Geometry: final body of the model. Coordinates: model frame, mm. A direction names the side the tool comes from. Give positions to 0.01 mm unless a question says otherwise; leave off trailing zeros. Order: outer loops, then holes, each group sorted by start corner. A loop starts at its lowest first (then second) coordinate and runs counter-clockwise, first axis right, second up. Notation, with made-up numbers: (39.5, 18) -> (44.5, 18) arc R7 cw to (44.5, 26) -> close; hole circle Ø10 at (-14, -27.5). An arc over 180 degrees is marked (long way). One line per question, with ' | ' between items.
from build123d import *

# Parameters (mm, degrees)
SKIZZE1_W                       = 64
SKIZZE1_H                       = 28
AUFSATZ_LINEAR_AUSTRAGEN1_DEPTH = 2
SKIZZE2_R                       = 1.75
SCHNITT_LINEAR_AUSTRAGEN1_DEPTH = 70.885620839
SKIZZE3_W                       = 2
SKIZZE3_H                       = 16
SCHNITT_LINEAR_AUSTRAGEN2_DEPTH = 70.885620839
LINEARES_MUSTER1_COUNT          = 4
LINEARES_MUSTER1_PITCH          = 4
SKIZZE5_W                       = 1.6
SKIZZE5_H                       = 10
SKIZZE5_W_2                     = 50
SKIZZE5_H_2                     = 1.6
SKIZZE5_W_3                     = 2
AUFSATZ_LINEAR_AUSTRAGEN2_DEPTH = 3
SKIZZE6_W                       = 52
SKIZZE6_H                       = 1.5
AUFSATZ_LINEAR_AUSTRAGEN3_DEPTH = 2
SKIZZE7_W                       = 56
SKIZZE7_H                       = 2.1
AUFSATZ_LINEAR_AUSTRAGEN4_DEPTH = 2
FASE1_SIZE2                     = 0.6
FASE1_SIZE                      = 2


with BuildPart() as part:
    # Skizze1 → Aufsatz-Linear austragen1 (new body)
    with BuildSketch(Plane(origin=(0, 0, 0), x_dir=(1, 0, 0), z_dir=(0, 1, 0))):
        with Locations((32, 14)):
            Rectangle(SKIZZE1_W, SKIZZE1_H)
    extrude(amount=AUFSATZ_LINEAR_AUSTRAGEN1_DEPTH)

    # Skizze2 → Schnitt-Linear austragen1 (cut, through all)
    with BuildSketch(Plane(origin=(0, 2, 0), x_dir=(1, 0, 0), z_dir=(0, 1, 0))):
        with Locations(Location((3, 3, 0), (0, 0, 270))):
            Circle(SKIZZE2_R)
        with Locations(Location((3, 20.9, 0), (0, 0, 270))):
            Circle(SKIZZE2_R)
        with Locations(Location((61, 20.9, 0), (0, 0, 270))):
            Circle(SKIZZE2_R)
        with Locations(Location((61, 3, 0), (0, 0, 270))):
            Circle(SKIZZE2_R)
    extrude(amount=-SCHNITT_LINEAR_AUSTRAGEN1_DEPTH, mode=Mode.SUBTRACT)

    # Skizze3 → Schnitt-Linear austragen2 (cut, through all)
    with BuildSketch(Plane(origin=(0, 2, 0), x_dir=(1, 0, 0), z_dir=(0, 1, 0))):
        with Locations((27, 14)):
            Rectangle(SKIZZE3_W, SKIZZE3_H)
    schnitt_linear_austragen2 = extrude(amount=-SCHNITT_LINEAR_AUSTRAGEN2_DEPTH, mode=Mode.SUBTRACT)

    # Lineares Muster1: Schnitt-Linear austragen2 ×4
    with Locations(*[(i * LINEARES_MUSTER1_PITCH, 0, 0) for i in range(1, LINEARES_MUSTER1_COUNT)]):
        add(schnitt_linear_austragen2, mode=Mode.SUBTRACT)

    # Skizze5 → Aufsatz-Linear austragen2 (add)
    with BuildSketch(Plane(origin=(0, 2, 0), x_dir=(1, 0, 0), z_dir=(0, 1, 0))):
        with Locations((2.8, 12)):
            Rectangle(SKIZZE5_W, SKIZZE5_H)
        with Locations((32, 2.8)):
            Rectangle(SKIZZE5_W_2, SKIZZE5_H_2)
        with Locations((61, 12)):
            Rectangle(SKIZZE5_W_3, SKIZZE5_H)
    extrude(amount=AUFSATZ_LINEAR_AUSTRAGEN2_DEPTH)

    # Skizze6 → Aufsatz-Linear austragen3 (add)
    with BuildSketch(Plane(origin=(0, 2, 0), x_dir=(1, 0, 0), z_dir=(0, 1, 0))):
        with Locations((32, 23.15)):
            Rectangle(SKIZZE6_W, SKIZZE6_H)
    extrude(amount=AUFSATZ_LINEAR_AUSTRAGEN3_DEPTH)

    # Skizze7 → Aufsatz-Linear austragen4 (add)
    with BuildSketch(Plane(origin=(0, 2, 0), x_dir=(1, 0, 0), z_dir=(0, 1, 0))):
        with Locations((32, 26.95)):
            Rectangle(SKIZZE7_W, SKIZZE7_H)
    extrude(amount=AUFSATZ_LINEAR_AUSTRAGEN4_DEPTH)

    # Fase1
    fase1_edges = [part.edges().sort_by_distance(p)[0] for p in [
        (32, 4, -25.9),
    ]]
    fase1_side = [part.faces().sort_by_distance(p)[0] for p in [
        (32, 3.988, -25.9),
    ]]
    chamfer(fase1_edges, length=FASE1_SIZE - 0.0001, length2=FASE1_SIZE2 - 0.0001, reference=fase1_side[0])  # a hair under: the kernel refuses the full size


solid = part.part
1) Section C-C on z = -20.9. Return loops of the section in (x, y), plus the area to 3 significant figures.
Check result:
outline: (0, 0) -> (1.25, 0) -> (1.25, 2) -> (0, 2) -> close; (4.75, 0) -> (26, 0) -> (26, 2) -> (4.75, 2) -> close; (28, 0) -> (30, 0) -> (30, 2) -> (28, 2) -> close; (32, 0) -> (34, 0) -> (34, 2) -> (32, 2) -> close; (36, 0) -> (38, 0) -> (38, 2) -> (36, 2) -> close; (40, 0) -> (59.25, 0) -> (59.25, 2) -> (40, 2) -> close; (62.75, 0) -> (64, 0) -> (64, 2) -> (62.75, 2) -> close | area: 98.0 mm^2
2) Material intervals for probe 1 along X at (y, z) = (1.35, -3); probe 2 along X at (y, z) = (1.85, -14); probe 3 along Z at (x, y) = (31, 2.5), sorted ascending. Write a range as from..to.
Check result:
probe 1: x = 0..1.25, 4.75..59.25, 62.75..64 | probe 2: x = 0..26, 28..30, 32..34, 36..38, 40..64 | probe 3: z = -28..-26.05, -23.9..-22.4, -3.6..-2
3) Section A-A on z = -9.5. Return loops of the section in (x, y).
Check result:
outline: (0, 0) -> (26, 0) -> (26, 2) -> (3.6, 2) -> (3.6, 5) -> (2, 5) -> (2, 2) -> (0, 2) -> close; (28, 0) -> (30, 0) -> (30, 2) -> (28, 2) -> close; (32, 0) -> (34, 0) -> (34, 2) -> (32, 2) -> close; (36, 0) -> (38, 0) -> (38, 2) -> (36, 2) -> close; (40, 0) -> (64, 0) -> (64, 2) -> (62, 2) -> (62, 5) -> (60, 5) -> (60, 2) -> (40, 2) -> close
4) Contact query for flat-ended pins moving along their axis: pin 1 Ø1.5 at (x, y) = (20.5, 3.5) entering from +Z; pin 2 Ø4.5 at (x, z) = (61, -3) entering from +Y; pin 3 Ø12 at (x, z) = (29, -15) entering from -Y; pin 4 Ø3 at (x, z) = (3, -20.9) entering from -Y. Output: stop coordinate, or through.
Check result:
pin 1: stops at z = -2 | pin 2: stops at y = 2 | pin 3: stops at y = 0 | pin 4: passes through
5) Section B-B on y = 1.1. Count the separate pieces of the cut face and the enclosed holes in it, plus the area to 3 significant figures.
Check result:
separate pieces: 1 | enclosed holes: 8 | area: 1,630 mm^2
6) Section D-D on x = 61. Return loops of the section in (y, z).
Check result:
outline: (0, -28) -> (2, -28) -> (2, -22.65) -> (0, -22.65) -> close; (0, -19.15) -> (2, -19.15) -> (2, -17) -> (5, -17) -> (5, -7) -> (2, -7) -> (2, -4.75) -> (0, -4.75) -> close; (0, -1.25) -> (2, -1.25) -> (2, 0) -> (0, 0) -> close
7) Pull-direction query (X, two-part tool) for faces 5 (the flat face through (2, 3, -12)), 6 (the flat face through (40, 1, -14)), 7 (the flat face through (31, 1, -6)), 8 (the flat face through (64, 1, -14)); classes: +X half, -X half, draft (parallel to the pull), parting line (faces both ways), or undercut.
Check result:
face 5: -X half | face 6: undercut | face 7: undercut | face 8: +X half
8) Set-up query: faces 1 (the flat face through (3.6, 3, -12)), 2 (the flat face through (32, 3, -22.4)), 3 (the flat face through (32, 4, -27)), 4 (the flat face through (36, 1, -14)). Return all of +Z, -Z, +X, -X, +Y, -Y with unobstructed straight access to the full face (end or side cutting, diameter ignored); none if empty.
Check result:
face 1: +Z, -Z, +Y | face 2: +X, -X, +Y | face 3: -Z, +X, -X, +Y | face 4: +Y, -Y
